Work out the finished part from the listing and answer in its coordinate system (mm). Round coordinates to 2 decimals unless told otherwise and drop trailing zeros. Write each loop counter-clockwise with the first axis right and the second up, starting at its lowest first coordinate (ties: lowest second). Pieces come first, ordered by that corner, then holes. Notation, with made-up numbers: (83, -27.5) - (113, -27.5) arc R20 ccw to (113, -22.5) - close; hole circle Ø11 at (2, 49). An arc over 180 degrees is marked (long way). Answer as a JSON object with one key per item and string values.
```python
from build123d import *

# Parameters (mm, degrees)
SKETCH_1_W          = 9
SKETCH_1_H          = 19
EXTRUDE_2_DEPTH     = 0.5
CUT_EXTRUDE_1_DEPTH = 53.98770037
FILLET_1_R          = 7


with BuildPart() as part:
    # 草圖1 → 填料-伸長2 (new body)
    with BuildSketch(Plane.XY):
        with Locations((4.5, 42.715384615)):
            Rectangle(SKETCH_1_W, SKETCH_1_H)
        with Locations((-4.5, 42.715384615)):
            Rectangle(SKETCH_1_W, SKETCH_1_H)
    extrude(amount=EXTRUDE_2_DEPTH)

    # 草圖3 → 除料-伸長1 (cut, through all)
    with BuildSketch(Plane.XY.offset(0.5)):
        with BuildLine():
            Line((0, 33.215384615), (9, 33.215384615))
            Line((9, 33.215384615), (9, 38.215384615))
            ThreePointArc((9, 38.215384615), (5.121083379, 34.597434532), (0, 33.215384615))
        make_face()
        with BuildLine():
            Line((-9, 33.215384615), (0, 33.215384615))
            ThreePointArc((0, 33.215384615), (-5.121083379, 34.597434532), (-9, 38.215384615))
            Line((-9, 38.215384615), (-9, 33.215384615))
        make_face()
    extrude(amount=-CUT_EXTRUDE_1_DEPTH, mode=Mode.SUBTRACT)

    # 圓角1
    fillet_1_edges = [part.edges().sort_by_distance(p)[0] for p in [
        (9, 38.215384615, 0.25),
        (-9, 38.215384615, 0.25),
    ]]
    fillet(fillet_1_edges, radius=FILLET_1_R)


solid = part.part
```
Item 1: A cutting plane is placed at C-C (x = -5.5). Write down the section's boundary in (y, z).
Results found:
{"outline": "(34.82, 0) - (52.22, 0) - (52.22, 0.5) - (34.82, 0.5) - close"}
Item 2: Consider line 1 along X through (y, z) = (34.75, 0.35); line 2 along Y through (x, z) = (-4, 0.45); line 3 along Y through (x, z) = (6.5, 0.2). Determine where each line is inside the solid, lowest interval first.
Results found:
{"line 1": "-5.39 to 5.39", "line 2": "34.06 to 52.22", "line 3": "35.52 to 52.22"}
Item 3: A cutting plane is placed at A-A (z = 0.1). Write down the section's boundary in (x, y).
Results found:
{"outline": "(-9, 40.89) arc R7 ccw to (-5.89, 35.06) arc R11 ccw to (0, 33.22) arc R11 ccw to (5.89, 35.06) arc R7 ccw to (9, 40.89) - (9, 52.22) - (-9, 52.22) - close"}
Item 4: A cutting plane is placed at B-B (y = 37.75). Write down the section's boundary in (x, z), and give its area (3 significant figures).
Results found:
{"outline": "(-8.26, 0) - (8.26, 0) - (8.26, 0.5) - (-8.26, 0.5) - close", "area": "8.26 mm²"}
